Source: CAD feature listing. Evaluate the final solid. Frame: model axes, mm. Round coordinates to 2 decimals unless told otherwise and drop trailing zeros. Loops run counter-clockwise (first coordinate to the right, second up) from the corner with the lowest first, then second, coordinate; pieces in that order, holes last. Notation, with made-up numbers: (3, 50) -> (19, 50) arc R28 cw to (19, 75) -> close; hole circle Ø3 at (57, 41). An arc over 180 degrees is marked (long way). Put each result on its own line as item: value. Start each with the question number.
1. Cut plane A-A (z = 0). Return the cut outline in (x, y) (3 decimals).
2. Material intervals for L1, parallel to Z at x = 0, y = 5 (3 decimals); L2, parallel to Z at x = -2, y = 0.75; L3, parallel to X at y = 7.75, z = 18.5, sorted ascending.
3. Cut plane B-B (x = 0). Return the cut outline in (y, z) (3 decimals).
4. Cut plane C-C (y = 1.5). State how many separate pieces and enclosed holes the cut face has, then the cut area to 3 significant figures.
5. Draft query along Z for faces 1 (the cylindrical face through (0.69, 4.7, 32.31)), 2 (the cylindrical face through (7.709, 4.383, 34.714)), 3 (the flat face through (0, 0, -23)). Return one class per face: pulls with the +Z half, pulls with the -Z half, needs draft (parallel to the pull), parting line crosses it, or undercut.
6. Contact query for flat-ended pins moving along their axis: pin 1 (5 mm diameter, centred on x = 26.5, y = 1.5, fed in from -Z); pin 2 (4 mm diameter, centred on x = -2, y = 6.5, fed in from +Z); pin 3 (3 mm diameter, centred on y = 5, z = 17.5, fed in from -X). Output: stop coordinate, or through.
Autodesk Inventor part; units mm, degrees
ref_plane "YZ Plane" through (0, 0, 0) normal (1, 0, 0) x (0, 1, 0)
ref_plane "XZ Plane" through (0, 0, 0) normal (0, 1, 0) x (-1, 0, 0)
ref_plane "XY Plane" through (0, 0, 0) normal (0, 0, 1) x (1, 0, 0)
sketch "Sketch1" plane through (0, 0, 0) normal (0, 1, 0) x (-1, 0, 0)
  circle A0 centre (0, 0) radius 35.56
  circle A1 centre (0, 0) radius 22.225
  line L0 (0, 0) -> (29.21, 0) construction
  circle A2 centre (29.21, 0) radius 3.175
  circle A3 centre (20.6546, 20.6546) radius 3.175
  circle A4 centre (0, 29.21) radius 3.175
  circle A5 centre (-20.6546, 20.6546) radius 3.175
  circle A6 centre (-29.21, 0) radius 3.175
  circle A7 centre (-20.6546, -20.6546) radius 3.175
  circle A8 centre (0, -29.21) radius 3.175
  circle A9 centre (20.6546, -20.6546) radius 3.175
  dimension "d0" = 71.12
  dimension "d1" = 44.45
  dimension "d2" = 29.21
  dimension "d3" = 6.35
  dimension "d6" = 360
extrude "Extrusion1" add sketch "Sketch1" along normal blind 9.525
thread "Thread1"
thread "Thread2"
thread "Thread3"
thread "Thread4"
thread "Thread5"
thread "Thread6"
thread "Thread7"
thread "Thread8"
chamfer "Chamfer1" distance 0.635 angle 45 2 edges at (35.56, 9.525, 0) (22.225, 9.525, 0)
equation "\"d2\" = 0.5 * d0 - d3"
properties part number "Rotary Pneumatic Cylinder Axis" material "Aluminum 6061"
Solution:
1. outline: (-35.56, 0) -> (-32.385, 0) -> (-32.385, 9.525) -> (-34.925, 9.525) -> (-35.56, 8.89) -> close; (-26.035, 0) -> (-22.225, 0) -> (-22.225, 8.89) -> (-22.86, 9.525) -> (-26.035, 9.525) -> close; (22.225, 0) -> (26.035, 0) -> (26.035, 9.525) -> (22.86, 9.525) -> (22.225, 8.89) -> close; (32.385, 0) -> (35.56, 0) -> (35.56, 8.89) -> (34.925, 9.525) -> (32.385, 9.525) -> close
2. L1: z = -35.56 to -32.385, -26.035 to -22.225, 22.225 to 26.035, 32.385 to 35.56
2. L2: z = -35.5 to -31.68, -26.74 to -22.13, 22.13 to 26.74, 31.68 to 35.5
2. L3: x = -30.37 to -22.99, -18.32 to -12.32, 12.32 to 18.32, 22.99 to 30.37
3. outline: (0, -35.56) -> (8.89, -35.56) -> (9.525, -34.925) -> (9.525, -32.385) -> (0, -32.385) -> close; (0, -26.035) -> (9.525, -26.035) -> (9.525, -22.86) -> (8.89, -22.225) -> (0, -22.225) -> close; (0, 22.225) -> (8.89, 22.225) -> (9.525, 22.86) -> (9.525, 26.035) -> (0, 26.035) -> close; (0, 32.385) -> (9.525, 32.385) -> (9.525, 34.925) -> (8.89, 35.56) -> (0, 35.56) -> close
4. separate pieces: 1
4. enclosed holes: 9
4. area: 2,170 mm^2
5. face 1: undercut
5. face 2: parting line crosses it
5. face 3: needs draft
6. pin 1: stops at z = -26.24
6. pin 2: stops at z = 35.56
6. pin 3: stops at x = -31.76
